Could you check a few things on this drawing? It's one solid part, dimensions in mm from its lowest x, y, z. A direction names the side the tool comes from. Round coordinates to 2 decimals unless told otherwise and drop trailing zeros. Loops run counter-clockwise (first coordinate to the right, second up) from the corner with the lowest first, then second, coordinate; pieces in that order, holes last. Notation, with made-up numbers: M -34,17 L 3,17 A33 cw 3,55 Z; hole C 41,24 d10. An arc over 180 degrees is marked long. Use a Markdown table: item, result. Add a question column.
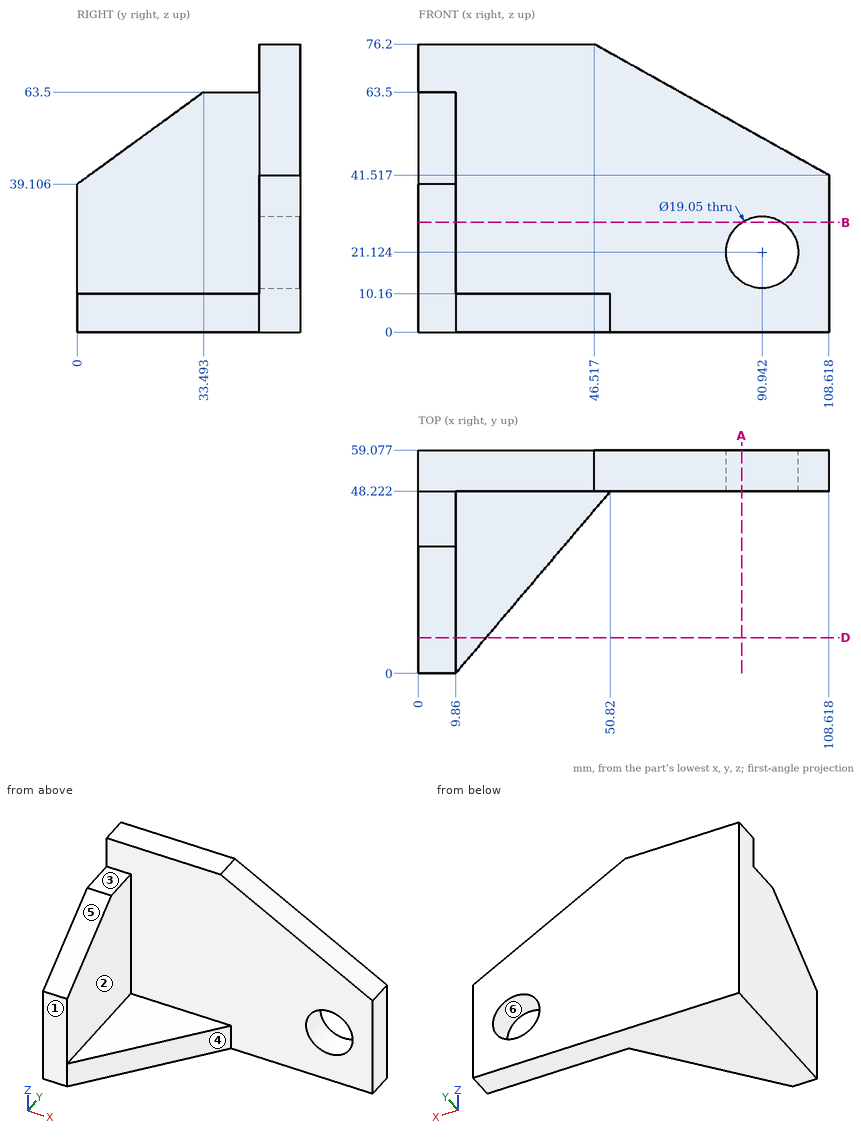
(1) I'm going to push flat-ended pins straight in: pin 1 (1.5 mm diameter, centred on x = 39, z = 50.5, fed in from -Y); pin 2 (20.5 mm diameter, centred on x = 38, y = 23, fed in from +Z); pin 3 (5 mm diameter, centred on x = 4.5, y = 41.5, fed in from +Z). Where does each tip first touch, or does it pass through?
(2) If I drill on probe 1 along X at (y, z) = (40, 16); probe 2 along Y at (x, z) = (25, 12.5); probe 3 along X at (y, z) = (54.5, 16), over which ranges is the centre line in solid material (lowest first)? Write a range as [from, to].
(3) Thinking about a two-plate mould opening in X: for the marked faces 4, 5 and 6, which applies, released by +X, released by -X, zero draft, split by the parting line, or undercut?
(4) Suppose I cut it at A-A on x = 85.5. List the corners of the cut face in (y, z) for me, and give its area (3 significant figures).
(5) Suppose I cut it at B-B on z = 29. List the corners of the cut face in (x, y) for me (1 decimal).
(6) On a 3-axis mill with a long thin cutter (end or side, diameter ignored), from which of +Z, -Z, +X, -X, +Y, -Y can I reach the whole of each face in a straight line? I mean the marked faces 1, 2 and 3. Say none if no direction works.
(7) Suppose I cut it at D-D on y = 9.5. List the corners of the cut face in (x, z) for me (1 decimal), and give its area (3 significant figures).
Results below:
| question | item | result |
|---|---|---|
| 1 | pin 1 | stops at y = 48.22 |
| 1 | pin 2 | stops at z = 10.16 |
| 1 | pin 3 | stops at z = 63.5 |
| 2 | probe 1 | x = [0, 9.86] |
| 2 | probe 2 | y = [48.22, 59.08] |
| 2 | probe 3 | x = [0, 82.91], [98.97, 108.62] |
| 3 | face 4 | released by +X |
| 3 | face 5 | zero draft |
| 3 | face 6 | undercut |
| 4 | outline | M 48.22,0 L 59.08,0 L 59.08,13.31 L 48.22,13.31 Z; M 48.22,28.94 L 59.08,28.94 L 59.08,54.43 L 48.22,54.43 Z |
| 4 | area | 421 mm² |
| 5 | outline | M 0,0 L 9.9,0 L 9.9,48.2 L 85.6,48.2 L 85.6,59.1 L 0,59.1 Z; M 96.3,48.2 L 108.6,48.2 L 108.6,59.1 L 96.3,59.1 Z |
| 6 | face 1 | +Z, -Z, +X, -X, -Y |
| 6 | face 2 | +Z, +X, -Y |
| 6 | face 3 | +Z, +X, -X, -Y |
| 7 | outline | M 0,0 L 17.9,0 L 17.9,10.2 L 9.9,10.2 L 9.9,46 L 0,46 Z |
| 7 | area | 536 mm² |
